from build123d import *

# Parameters (mm, degrees)
SKETCH1_W           = 88
SKETCH1_H           = 56
BOSS_EXTRUDE1_DEPTH = 9
BOSS_EXTRUDE2_DEPTH = 34
SKETCH3_W           = 14
SKETCH3_H           = 24
CUT_EXTRUDE1_DEPTH  = 103.703456612


with BuildPart() as part:
    # Sketch1 → Boss-Extrude1 (new body)
    with BuildSketch(Plane(origin=(0, 0, 0), x_dir=(1, 0, 0), z_dir=(0, 1, 0))):
        Rectangle(SKETCH1_W, SKETCH1_H)
    extrude(amount=BOSS_EXTRUDE1_DEPTH)

    # Sketch2 → Boss-Extrude2 (add)
    with BuildSketch(Plane.XY.offset(17)):
        Polygon((-44, 9), (36, 9), (36, 58), (10, 58), (-44, 26), align=None)
    extrude(amount=-BOSS_EXTRUDE2_DEPTH)

    # Sketch3 → Cut-Extrude1 (cut, through all)
    with BuildSketch(Plane(origin=(36, 0, 0), x_dir=(0, 0, -1), z_dir=(1, 0, 0))):
        with Locations((0, 42.74)):
            Rectangle(SKETCH3_W, SKETCH3_H)
    extrude(amount=-CUT_EXTRUDE1_DEPTH, mode=Mode.SUBTRACT)


solid = part.part
Verification items for the finished model (mm, model axes). A direction names the side the tool comes from. Round coordinates to 2 decimals unless told otherwise and drop trailing zeros. Loops run counter-clockwise (first coordinate to the right, second up) from the corner with the lowest first, then second, coordinate; pieces in that order, holes last. Notation, with made-up numbers: M 34,40.5 L 82,40.5 A30 ccw 82,62.5 Z; hole C -19,87.25 d7. An arc over 180 degrees is marked long. Write each question's results on one line, items separated by ' | '.
1) Gauge pin test, flat ends, axial feed: P1, Ø1, axis at x = -12.5, z = -11.5, coming from the +Y side; P2, Ø5, axis at x = -20, y = 15, coming from the +Z side; P3, Ø7, axis at x = -16, z = -2.5, coming from the +Y side. Record the tip position at first contact, or that the pin passes through.
Checks:
P1: stops at y = 44.96 | P2: stops at z = 17 | P3: stops at y = 30.74
2) Scan lines: L1, parallel to Z at x = -20, y = 39; L2, parallel to Y at x = 16, z = -6; L3, parallel to Y at x = 24.5, z = 24.5. Record each from-to range of solid material in increasing order. Write a range as from..to.
Checks:
L1: z = -17..-7, 7..17 | L2: y = 0..30.74, 54.74..58 | L3: y = 0..9
3) Section check A-A on x = 13.5. Record the boundary of the cut face in (y, z).
Checks:
outline: M 0,-28 L 9,-28 L 9,-17 L 58,-17 L 58,17 L 9,17 L 9,28 L 0,28 Z; hole M 30.74,-7 L 54.74,-7 L 54.74,7 L 30.74,7 Z
4) Section check D-D on z = -10. Record the boundary of the cut face in (x, y).
Checks:
outline: M -44,0 L 44,0 L 44,9 L 36,9 L 36,58 L 10,58 L -44,26 Z
5) Access from +Z, -Z, +X, -X, +Y, -Y to the whole of each face (thin tool, end or side, straight path). Record for faces 4 (the flat face through (36, 28, 0)), 5 (the flat face through (-1, 4, 28)), 6 (the flat face through (20, 54.74, 0)), 7 (the flat face through (4, 28, 17)), 8 (the flat face through (4, 28, -17)).
Checks:
face 4: +Z, -Z, +X, +Y | face 5: +Z, +X, -X, +Y, -Y | face 6: +X, -X | face 7: +Z, +X, -X, +Y | face 8: -Z, +X, -X, +Y
6) Mould release check, pull along Z, two halves, no side actions. Record for faces 1 (the flat face through (-1, 4, -28)), 2 (the flat face through (9, 40, 7)), 3 (the flat face through (44, 4, 0)): released by +Z, released by -Z, zero draft, split by the parting line, or undercut.
Checks:
face 1: released by -Z | face 2: undercut | face 3: zero draft
7) Section check B-B on z = 1. Record the boundary of the cut face in (x, y), then the cut area to 3 significant figures.
Checks:
outline: M -44,0 L 44,0 L 44,9 L 36,9 L 36,30.74 L -36,30.74 L -44,26 Z; M 4.5,54.74 L 36,54.74 L 36,58 L 10,58 Z | area: 2,610 mm2
8) Section check C-C on y = 41. Record the boundary of the cut face in (x, z).
Checks:
outline: M -18.69,-17 L 36,-17 L 36,-7 L -18.69,-7 Z; M -18.69,7 L 36,7 L 36,17 L -18.69,17 Z
